Input: part model. Units: mm. Frame: model coordinates. Face numbers are marked on the shaded views. Coordinates: 2 decimals unless noted, no trailing zeros. Write each loop counter-clockwise with the first axis right and the second up, starting at its lowest first coordinate (ties: lowest second). Pieces come first, ordered by that corner, then holes. Notation, with made-up numbers: (-26.75, 4.25) -> (22.25, 4.25) arc R26 ccw to (22.25, 40.25) -> close; hole circle Ø3 at (83, 51). An arc over 180 degrees is marked (long way). Use one line per item in the form item = value. Start each with the question number.
(1) Cut plane A-A on x = 0. Return the cut outline in (y, z), plus the area to 3 significant figures.
(2) Pull-direction query (X, two-part tool) for the marked faces 1, 2 and 3; classes: released by +X, released by -X, zero draft, split by the parting line, or undercut.
(3) Ray query, line 1 along Y through (x, z) = (-53.5, 76); line 2 along Y through (x, z) = (-61, 92); line 3 along X through (y, z) = (0, 58.5). Return the intervals inside material, ascending.
(4) Cut plane C-C on z = 82. Return the cut outline in (x, y).
(5) First-contact query: pin 1 (1.5 mm diameter, centred on x = 40.5, y = -46.5, fed in from -Z); pin 2 (11 mm diameter, centred on x = 58.34, y = 58.34, fed in from -Z). Flat tips, straight axial feed; report the tip coordinate or a pass-through.
(6) Cut plane D-D on y = -56. Return the cut outline in (x, z).
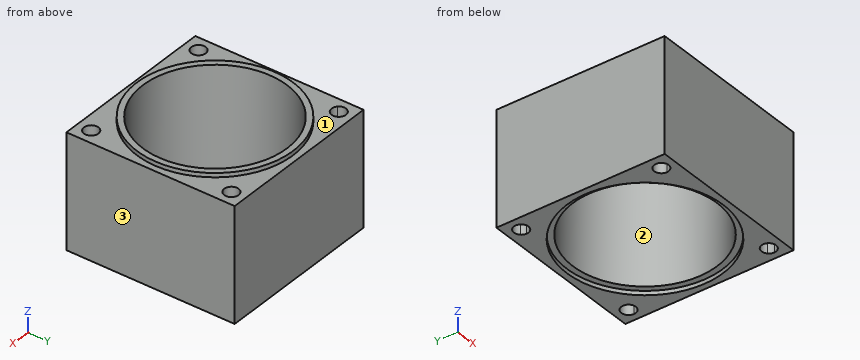
```python
from build123d import *

# Parameters (mm, degrees)
F0_W     = 140
F0_H     = 140
F0_R     = 60
F1_DEPTH = 95
F2_R     = 65
F2_R_2   = 60
F3_DEPTH = 3.5
F4_R     = 65
F4_R_2   = 50
F5_DEPTH = 3.5
F7_DEPTH = 95.001


with BuildPart() as f1:
    # F0 (on Top) → F1 (new body)
    with BuildSketch(Plane.XY):
        Rectangle(F0_W, F0_H)
        Circle(F0_R, mode=Mode.SUBTRACT)
    extrude(amount=F1_DEPTH)

    # F2 (on face) → F3 (join)
    with BuildSketch(Plane.XY.offset(95)):
        Circle(F2_R)
        Circle(F2_R_2, mode=Mode.SUBTRACT)
    extrude(amount=F3_DEPTH)

    # F4 (on face) → F5 (cut)
    with BuildSketch(Plane(origin=(0, 0, 0), x_dir=(1, 0, 0), z_dir=(0, 0, -1))):
        Circle(F4_R)
        Circle(F4_R_2, mode=Mode.SUBTRACT)
    extrude(amount=-F5_DEPTH, mode=Mode.SUBTRACT)

    # F6 (on face) → F7 (cut, through all)
    with BuildSketch(Plane.XY.offset(95)):
        with BuildLine():
            ThreePointArc((-58.3363094479, 58.3363094479), (-56.1764068849, 60.419047572), (-53.9421968972, 62.4218663122))
            ThreePointArc((-53.9421968972, 62.4218663122), (-58.2272004968, 64.3353173023), (-62.578950135, 62.578950135))
            Line((-62.578950135, 62.578950135), (-58.3363094479, 58.3363094479))
        make_face()
        with BuildLine():
            ThreePointArc((-52.3363094479, 58.3363094479), (-52.752194688, 60.5312268377), (-53.9421968972, 62.4218663122))
            ThreePointArc((-53.9421968972, 62.4218663122), (-56.1764068849, 60.419047572), (-58.3363094479, 58.3363094479))
            Line((-58.3363094479, 58.3363094479), (-54.0936687608, 54.0936687608))
            ThreePointArc((-54.0936687608, 54.0936687608), (-52.7930322528, 56.0402088537), (-52.3363094479, 58.3363094479))
        make_face()
        with BuildLine():
            Line((-54.0936687608, 54.0936687608), (-58.3363094479, 58.3363094479))
            ThreePointArc((-58.3363094479, 58.3363094479), (-60.419047572, 56.1764068849), (-62.4218663122, 53.9421968972))
            ThreePointArc((-62.4218663122, 53.9421968972), (-58.2272004968, 52.3373015935), (-54.0936687608, 54.0936687608))
        make_face()
        with BuildLine():
            ThreePointArc((-62.4218663122, 53.9421968972), (-60.419047572, 56.1764068849), (-58.3363094479, 58.3363094479))
            Line((-58.3363094479, 58.3363094479), (-62.578950135, 62.578950135))
            ThreePointArc((-62.578950135, 62.578950135), (-64.3353173023, 58.2272004968), (-62.4218663122, 53.9421968972))
        make_face()
        with BuildLine():
            ThreePointArc((53.9421968972, 62.4218663122), (58.3363094479, 58.3363094479), (62.4218663122, 53.9421968972))
            ThreePointArc((62.4218663122, 53.9421968972), (63.836915832, 55.9397850047), (64.3363094479, 58.3363094479))
            ThreePointArc((64.3363094479, 58.3363094479), (60.5312268377, 63.9204242078), (53.9421968972, 62.4218663122))
        make_face()
        with BuildLine():
            ThreePointArc((53.9421968972, 62.4218663122), (54.0936687608, 54.0936687608), (62.4218663122, 53.9421968972))
            ThreePointArc((62.4218663122, 53.9421968972), (58.3363094479, 58.3363094479), (53.9421968972, 62.4218663122))
        make_face()
        with BuildLine():
            ThreePointArc((64.3363094479, -58.3363094479), (63.836915832, -55.9397850047), (62.4218663122, -53.9421968972))
            ThreePointArc((62.4218663122, -53.9421968972), (58.3363094479, -58.3363094479), (53.9421968972, -62.4218663122))
            ThreePointArc((53.9421968972, -62.4218663122), (60.5312268377, -63.9204242078), (64.3363094479, -58.3363094479))
        make_face()
        with BuildLine():
            ThreePointArc((53.9421968972, -62.4218663122), (58.3363094479, -58.3363094479), (62.4218663122, -53.9421968972))
            ThreePointArc((62.4218663122, -53.9421968972), (54.0936687608, -54.0936687608), (53.9421968972, -62.4218663122))
        make_face()
        with BuildLine():
            ThreePointArc((-62.4218663122, -53.9421968972), (-62.578950135, -62.578950135), (-53.9421968972, -62.4218663122))
            ThreePointArc((-53.9421968972, -62.4218663122), (-58.3363094479, -58.3363094479), (-62.4218663122, -53.9421968972))
        make_face()
        with BuildLine():
            ThreePointArc((-62.4218663122, -53.9421968972), (-58.3363094479, -58.3363094479), (-53.9421968972, -62.4218663122))
            ThreePointArc((-53.9421968972, -62.4218663122), (-52.752194688, -60.5312268377), (-52.3363094479, -58.3363094479))
            ThreePointArc((-52.3363094479, -58.3363094479), (-55.9397850047, -52.8357030638), (-62.4218663122, -53.9421968972))
        make_face()
    extrude(amount=-F7_DEPTH, mode=Mode.SUBTRACT)


solid = f1.part
```
Values:
q1.outline = (-70, 0) -> (-65, 0) -> (-65, 3.5) -> (-60, 3.5) -> (-60, 98.5) -> (-65, 98.5) -> (-65, 95) -> (-70, 95) -> close; (60, 3.5) -> (65, 3.5) -> (65, 0) -> (70, 0) -> (70, 95) -> (65, 95) -> (65, 98.5) -> (60, 98.5) -> close
q1.area = 1,900 mm2
q2.face_1 = zero draft
q2.face_2 = undercut
q2.face_3 = released by +X
q3.line_1 = -70 to -61.89, -54.79 to -27.16, 27.16 to 54.79, 61.89 to 70
q3.line_2 = -70 to -63.71, -52.96 to 52.96, 63.71 to 70
q3.line_3 = -70 to -60, 60 to 70
q4.outline = (-70, -70) -> (70, -70) -> (70, 70) -> (-70, 70) -> close; hole circle Ø12 at (-58.34, -58.34); hole circle Ø12 at (-58.34, 58.34); hole circle Ø120 at (0, 0); hole circle Ø12 at (58.34, -58.34); hole circle Ø12 at (58.34, 58.34)
q5.pin_1 = 3.5
q5.pin_2 = through
q6.outline = (-70, 0) -> (-63.86, 0) -> (-63.86, 95) -> (-70, 95) -> close; (-52.81, 0) -> (-33, 0) -> (-33, 3.5) -> (-21.54, 3.5) -> (-21.54, 98.5) -> (-33, 98.5) -> (-33, 95) -> (-52.81, 95) -> close; (21.54, 3.5) -> (33, 3.5) -> (33, 0) -> (52.81, 0) -> (52.81, 95) -> (33, 95) -> (33, 98.5) -> (21.54, 98.5) -> close; (63.86, 0) -> (70, 0) -> (70, 95) -> (63.86, 95) -> close
